Autodesk Inventor part; units mm, degrees
ref_plane "YZ Plane" through (0, 0, 0) normal (1, 0, 0) x (0, 1, 0)
ref_plane "XZ Plane" through (0, 0, 0) normal (0, 1, 0) x (-1, 0, 0)
ref_plane "XY Plane" through (0, 0, 0) normal (0, 0, 1) x (1, 0, 0)
sketch "草圖1" plane through (0, 0, 0) normal (0, 1, 0) x (-1, 0, 0)
  line L0 (10, 15) -> (-15, 15)
  line L1 (-15, 15) -> (-15, 5)
  line L2 (-10, 0) -> (0, 0)
  line L3 (10, 0) -> (10, 15)
  line L4 (10, 15) -> (0, 15)
  line L5 (0, 0) -> (0, -10)
  line L6 (5, -15) -> (10, -15)
  line L7 (10, -15) -> (10, 15)
  arc A0 (0, -10) -> (5, -15) centre (5, -10) ccw
  arc A1 (-15, 5) -> (-10, 0) centre (-10, 5) ccw
  point P0 (-15, 0)
  point P1 (0, -15)
  dimension "d0" = 15
  dimension "d1" = 10
  dimension "d2" = 30
  dimension "d3" = 25
  dimension "d4" = 5
extrude "擠出1" add sketch "草圖1" along normal blind 5
sketch "草圖2" plane through (-10, 0, -15) normal (-1, 0, 0) x (0, 0, 1)
  line L0 (30, 0) -> (20, 0) construction
  line L1 (20, 0) -> (20, 5) construction
  line L2 (30, 5) -> (20, 5) construction
  line L3 (30, 0) -> (30, 5) construction
  line L4 (20, 0) -> (15, 0) construction
  line L5 (15, 0) -> (15, 5) construction
  line L6 (20, 5) -> (15, 5) construction
  line L7 (20, 0) -> (20, 5) construction
  line L8 (15, 0) -> (5, 0) construction
  line L9 (5, 0) -> (5, 5) construction
  line L10 (15, 5) -> (5, 5) construction
  line L11 (15, 0) -> (15, 5) construction
  line L12 (5, 0) -> (0, 0) construction
  line L13 (0, 0) -> (0, 5) construction
  line L14 (5, 5) -> (0, 5) construction
  line L15 (5, 0) -> (5, 5) construction
  line L16 (30, 0) -> (30, 5)
  line L17 (30, 5) -> (20, 5)
  line L18 (20, 10) -> (20, 15)
  line L19 (20, 15) -> (30, 15)
  line L20 (30, 15) -> (30, 5)
  line L21 (15, 5) -> (5, 5)
  line L22 (20, 10) -> (5, 10)
  line L23 (5, 5) -> (20, 5)
  line L24 (0, 5) -> (30, 5)
  line L25 (0, 5) -> (5, 5)
  line L26 (5, 10) -> (5, 25)
  line L27 (5, 25) -> (5, 25)
  line L28 (0, 20) -> (0, 5)
  arc A0 (5, 25) -> (0, 20) centre (5, 20) ccw
  point P0 (0, 25)
  dimension "d7" = 5
  dimension "d8" = 10
  dimension "d9" = 10
  dimension "d10" = 5
  dimension "d11" = 20
  dimension "d12" = 5
extrude "擠出2" add sketch "草圖2" against normal blind 5
sketch "草圖3" plane through (-10, 0, 15) normal (0, 0, 1) x (1, 0, 0)
  line L0 (0, 0) -> (25, 0) construction
  line L1 (25, 0) -> (25, 5) construction
  line L2 (5, 5) -> (25, 5) construction
  line L3 (5, 15) -> (5, 5) construction
  line L4 (0, 15) -> (5, 15) construction
  line L5 (0, 0) -> (0, 15) construction
  line L6 (5, 5) -> (25, 5)
  line L7 (5, 15) -> (25, 5)
  line L8 (25, 5) -> (5, 5)
  line L9 (5, 5) -> (5, 15)
  point P0 (10, 0)
extrude "擠出3" add sketch "草圖3" against normal blind 5
properties part number "5"
Could you check a few things on this model? Use its own coordinates, in mm. A direction names the side the tool comes from. Round coordinates to 2 decimals unless told otherwise and drop trailing zeros. Loops run counter-clockwise (first coordinate to the right, second up) from the corner with the lowest first, then second, coordinate; pieces in that order, holes last. Notation, with made-up numbers: (24, -5.75) - (62, -5.75) arc R21 cw to (62, 22.25) - close; hole circle Ø11 at (63, 68). An arc over 180 degrees is marked (long way). Write item = value, one per line.
1) Imagine slicing it at B-B (y = 2). Please give me the cut outline in (x, z).
Computed:
outline = (-10, -15) - (-5, -15) arc R5 ccw to (0, -10) - (0, 0) - (10, 0) arc R5 ccw to (15, 5) - (15, 15) - (-10, 15) - close
2) On a 3-axis mill with a long thin cutter (end or side, diameter ignored), from which of +Z, -Z, +X, -X, +Y, -Y can I reach the whole of each face in a straight line? I mean faces 4 (the flat face through (-8, 15, 10)), 5 (the flat face through (0, 2, -5)), 6 (the flat face through (-5, 8, -5)), 7 (the flat face through (-8, 12, 5)). Say none if no direction works.
Computed:
face_4 = +Z, +X, -X, +Y
face_5 = -Z, +X, +Y, -Y
face_6 = -Z, +X, +Y
face_7 = +X, -X, +Y
3) If we mould it in two halves opening along Z, with no side actions, what happens to faces 1 (the flat face through (-8, 10, -2)), 2 (the flat face through (5, 2, 0)), 3 (the flat face through (15, 2, 10))? For each: pulls with the +Z half, pulls with the -Z half, needs draft (parallel to the pull), parting line crosses it, or undercut.
Computed:
face_1 = undercut
face_2 = pulls with the -Z half
face_3 = needs draft
4) Imagine slicing it at D-D (z = -6). Please give me the cut outline in (x, y), and give its area (3 significant figures).
Computed:
outline = (-10, 0) - (0, 0) - (0, 5) - (-5, 5) - (-5, 10) - (-10, 10) - close
area = 75.0 mm2
5) Imagine slicing it at C-C (x = -7). Please give me the cut outline in (y, z), and give its area (3 significant figures).
Computed:
outline = (0, -15) - (20, -15) arc R5 ccw to (25, -10) - (10, -10) - (10, 5) - (15, 5) - (15, 15) - (0, 15) - close
area = 420 mm2
6) I need wall thicknesses on line 1 along X through (y, z) = (18.75, -13.5); line 2 along Y through (x, z) = (10, 0.5); line 3 along Z through (x, y) = (0, 10.5). Which ranges of each line are inside material? Lowest first, please. Write a range as from..to.
Computed:
line_1 = -10..-5
line_2 = 0..5
line_3 = 10..15
7) I'm going to push flat-ended pins straight in: P1, Ø2.5, axis at x = -8, z = 11, coming from the +Y side; P2, Ø10, axis at y = 15.5, z = -8, coming from the +X side; P3, Ø12, axis at x = 5, z = -2.5, coming from the -Y side; P4, Ø1.5, axis at x = 3.5, y = 2.5, coming from the -Z side. Where does each tip first touch, or does it pass through?
Computed:
P1 = 15
P2 = -5
P3 = 0
P4 = 0
8) Imagine slicing it at A-A (y = 12.25). Please give me the cut outline in (x, z).
Computed:
outline = (-10, -15) - (-5, -15) - (-5, -10) - (-10, -10) - close; (-10, 5) - (-5, 5) - (-5, 10) - (0.5, 10) - (0.5, 15) - (-10, 15) - close
